Part model, mm, in its own coordinate system. A direction names the side the tool comes from. Coordinates: 2 decimals unless noted, no trailing zeros. Write each loop counter-clockwise with the first axis right and the second up, starting at its lowest first coordinate (ties: lowest second). Pieces come first, ordered by that corner, then holes. Notation, with made-up numbers: (51, 19) - (87, 19) arc R21 ccw to (87, 49) - close; hole circle Ø3 at (49.25, -39.75). An arc over 180 degrees is marked (long way). Use one line per item in the form item = value. Start each with the question number.
from build123d import *

# Parameters (mm, degrees)
SKETCH_1_R           = 2.4
EXTRUDE_1_DEPTH      = 2.1
EXTRUDE_START        = 1
SKETCH_1_9_R         = 11.65
SKETCH_1_9_R_2       = 2.4
EXTRUDE_2_DEPTH      = 1
EXTRUDE_3_DEPTH      = 1
EXTRUDE_3_DEPTH_BACK = 2.1
SKETCH_1_10_R        = 12.65
SKETCH_1_10_R_2      = 11.65
FILLET_1_R           = 1
FILLET_2_R           = 0.5
FILLET_3_R           = 0.5
FILLET_4_R           = 1


with BuildPart() as part:
    # 草图1 → 凸台-拉伸1 (new body)
    with BuildSketch(Plane.XY):
        Circle(SKETCH_1_R)
        Polygon((0.55, -2), (0.55, -0.55), (2, -0.55), (2, 0.55), (0.55, 0.55), (0.55, 2), (-0.55, 2), (-0.55, 0.55), (-2, 0.55), (-2, -0.55), (-0.55, -0.55), (-0.55, -2), align=None, mode=Mode.SUBTRACT)
    extrude(amount=-EXTRUDE_1_DEPTH)

    # 草图1<9> → 凸台-拉伸2 (add)
    # profile 1 of 3: a face of its own
    with BuildSketch(Plane.XY.offset(EXTRUDE_START)):
        Circle(SKETCH_1_9_R)
        Circle(SKETCH_1_9_R_2, mode=Mode.SUBTRACT)
    # profile 2 of 3: a face of its own
    with BuildSketch(Plane.XY.offset(EXTRUDE_START)):
        Circle(SKETCH_1_9_R_2)
        Polygon((0.55, -2), (0.55, -0.55), (2, -0.55), (2, 0.55), (0.55, 0.55), (0.55, 2), (-0.55, 2), (-0.55, 0.55), (-2, 0.55), (-2, -0.55), (-0.55, -0.55), (-0.55, -2), align=None, mode=Mode.SUBTRACT)
    # profile 3 of 3: a face of its own
    with BuildSketch(Plane.XY.offset(EXTRUDE_START)):
        Polygon((-0.55, -2), (0.55, -2), (0.55, -0.55), (2, -0.55), (2, 0.55), (0.55, 0.55), (0.55, 2), (-0.55, 2), (-0.55, 0.55), (-2, 0.55), (-2, -0.55), (-0.55, -0.55), align=None)
    extrude(amount=-EXTRUDE_2_DEPTH)

    # 草图1<10> → 凸台-拉伸3 (add, two sides: drawn at the far end of the back side and taken through both)
    with BuildSketch(Plane.XY.offset(-EXTRUDE_3_DEPTH_BACK)):
        Circle(SKETCH_1_10_R)
        Circle(SKETCH_1_10_R_2, mode=Mode.SUBTRACT)
    extrude(amount=EXTRUDE_3_DEPTH + EXTRUDE_3_DEPTH_BACK)

    # 圆角1
    fillet_1_edges = [part.edges().sort_by_distance(p)[0] for p in [
        (-12.65, 0, 1),
    ]]
    fillet(fillet_1_edges, radius=FILLET_1_R - 0.0001)  # a hair under: the kernel refuses the full size

    # 圆角2
    fillet_2_edges = [part.edges().sort_by_distance(p)[0] for p in [
        (-11.65, 0, -2.1),
    ]]
    fillet(fillet_2_edges, radius=FILLET_2_R)

    # 圆角3
    fillet_3_edges = [part.edges().sort_by_distance(p)[0] for p in [
        (-12.65, 0, -2.1),
    ]]
    fillet(fillet_3_edges, radius=FILLET_3_R - 0.0001)  # a hair under: the kernel refuses the full size

    # 圆角4
    fillet_4_edges = [part.edges().sort_by_distance(p)[0] for p in [
        (-11.65, 0, 0),
    ]]
    fillet(fillet_4_edges, radius=FILLET_4_R)


solid = part.part
Q1. Drill centre lines: probe 1 along Y at (x, z) = (0, -1.5); probe 2 along X at (y, z) = (1.25, -0.25); probe 3 along Y at (x, z) = (0.5, -1.25). Where is each one in solid material? Low to high.
Q2. Which spindle directions (+Z, -Z, +X, -X, +Y, -Y) get a long thin tool onto all of the face, cutting with end or side? Do faces 1 (the cylindrical face through (1.29, 2.024, -1.035)), 2 (the flat face through (-1, 1, -2.1)). Say none if no direction does.
Q3. Mould opens along Y. For faces 3 (the flat face through (0, 0, 1)), 4 (the cylindrical face through (-2.74, -12.35, -0.81)), 5 (the flat face through (-0.55, -1, -1)) say: released by +Y, released by -Y, zero draft, split by the parting line, or undercut.
Q4. Pin check, flat tips, straight feed: P1, Ø0.7, axis at y = 1, z = -1, coming from the -X side; P2, Ø1.6, axis at x = -1.5, z = -0.5, coming from the -Y side; P3, Ø1, axis at y = 5.5, z = -1.5, coming from the -X side. Stop position of each tip, or through.
Q5. Slice it at C-C (z = 0.5). List the corners of the cut face in (x, y).
Solution:
q1.probe_1 = -12.65 to -11.65, -2.4 to -2, 2 to 2.4, 11.65 to 12.65
q1.probe_2 = -12.59 to -11.24, -2.05 to -0.55, 0.55 to 2.05, 11.24 to 12.59
q1.probe_3 = -12.64 to -11.64, -2.35 to -2, 2 to 2.35, 11.64 to 12.64
q2.face_1 = -Z
q2.face_2 = -Z, +X, -X, +Y, -Y
q3.face_3 = zero draft
q3.face_4 = split by the parting line
q3.face_5 = undercut
q4.P1 = -12.63
q4.P2 = -12.63
q4.P3 = -11.62
q5.outline = circle Ø25.03 at (0, 0)
